Can you work these out from the model? Positions are in its coordinate system, mm. Give positions to 0.01 mm unless a question says otherwise; leave off trailing zeros. Order: outer loops, then holes, each group sorted by start corner. A loop starts at its lowest first (then second) coordinate and runs counter-clockwise, first axis right, second up. Notation, with made-up numbers: M 42.5,-25.75 L 48.5,-25.75 A38 cw 48.5,13.25 Z; hole C 41,66 d11. An arc over 180 degrees is marked long. One line per question, with ' | ' between items. Start each with the question number.
1) If we section it at A-A, the plane x = 0: Please give me the cut outline in (y, z).
2) I'm going to push flat-ended pins straight in: pin 1 Ø2 at (x, z) = (24.5, -180) entering from -Y; pin 2 Ø1.5 at (x, y) = (-2.5, 82) entering from -Z; pin 3 Ø12 at (x, y) = (24, -4) entering from +Z. Where does each tip first touch, or does it pass through?
3) If we section it at C-C, the plane y = -13.5: Please give me the cut outline in (x, z), plus the area to 3 significant figures.
4) Please list where these lines run through material, in increasing order: line 1 along Y through (x, z) = (11.5, -65) (3 decimals); line 2 along Y through (x, z) = (-6, -88); line 3 along Z through (x, y) = (5.5, 12). Write a range as [from, to].
5) If we section it at B-B, the plane z = -207.5: Please give me the cut outline in (x, y), plus the area to 3 significant figures.
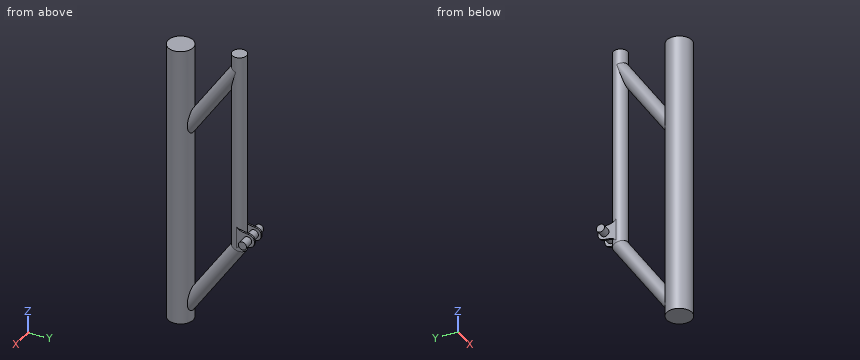
```python
from build123d import *

# Parameters (mm, degrees)
SKETCH1_R                = 25.8
BOSS_EXTRUDE1_DEPTH      = 544
SKETCH6_R                = 14.6
BOSS_EXTRUDE2_REACH      = 541.822
BOSS_EXTRUDE2_END_RADIUS = 25.8
SKETCH4_R                = 14.6
BOSS_EXTRUDE3_START      = -3.5
BOSS_EXTRUDE3_OUTLINE_R  = 8.35
BOSS_EXTRUDE3_DEPTH      = 3.5
BOSS_EXTRUDE4_START      = 17
SKETCH7_3_R              = 8.35
BOSS_EXTRUDE4_DEPTH      = 66
SKETCH9_R                = 25.8
BOSS_EXTRUDE5_DEPTH      = 16.49
BOSS_EXTRUDE6_START      = 23.51
SKETCH10_R               = 25.8
BOSS_EXTRUDE6_DEPTH      = 23.51
BOSS_EXTRUDE7_START      = 13
SKETCH11_R               = 14.6
BOSS_EXTRUDE7_DEPTH      = 13


# Read off the part's stored shape, not the designer's step: Boss-Extrude3
with BuildPart() as part:
    # Sketch1 → Boss-Extrude1 (new body)
    with BuildSketch(Plane.XY):
        Circle(SKETCH1_R)
    extrude(amount=-BOSS_EXTRUDE1_DEPTH)

    # Sweep2: sweep along a path in Sketch2
    with BuildLine(Plane(origin=(0, 0, 0), x_dir=(0, 0, -1), z_dir=(1, 0, 0))) as sweep2_path:
        Line((535.242725219, 10.616416132), (373.485286901, 119.6))
        Line((373.485286901, 119.6), (-26.514713099, 119.6))
    # Sketch6 → Sweep2 (sweep)
    with BuildSketch(Plane(origin=(0, 10.616416132, -535.242725219), x_dir=(1, 0, 0), z_dir=(0, 0.5587587437797145, 0.8293302516185669))):
        Circle(SKETCH6_R)
    sweep(path=sweep2_path.line, transition=Transition.RIGHT)

    # Boss-Extrude2: up to this cylinder (the profile starts outside it)
    boss_extrude2_end = Plane(origin=(0, 0, 7.489761), z_dir=(0, 0, 1)) * Cylinder(BOSS_EXTRUDE2_END_RADIUS, 1136.244, mode=Mode.PRIVATE)
    # Sketch4 → Boss-Extrude2 (add, up to the surface)
    with BuildSketch(Plane(origin=(0, 296.142134203, -111.454966642), x_dir=(1, 0, 0), z_dir=(0, 0.5587587437797145, 0.8293302516185669)), mode=Mode.PRIVATE) as boss_extrude2_sk1:
        with Locations(Location((0, -212.87313933, 0), (0, 0, 270))):
            Circle(SKETCH4_R)
    boss_extrude2_tool1 = extrude(boss_extrude2_sk1.sketch, amount=-BOSS_EXTRUDE2_REACH, mode=Mode.PRIVATE) - boss_extrude2_end
    add(boss_extrude2_tool1.solids().sort_by_distance((0, 119.6, 7.489761))[0])

    # Boss-Extrude3 outline → Boss-Extrude3 (add)
    with BuildSketch(Plane.ZY.offset(14.6).offset(BOSS_EXTRUDE3_START)):
        with BuildLine():
            add(Edge.make_bspline(
                [(-369.025798161, 121.314868638), (-354.153662916, 130.263805611), (-368.24558028, 157.483504956), (-346.0257981, 157.599948143)],
                knots=[0, 0, 0, 0, 0.999846057, 0.999846057, 0.999846057, 0.999846057], degree=3))
            Line((-369.025798161, 121.314868638), (-323.025798161, 121.314868638))
            add(Edge.make_bspline(
                [(-323.025798161, 121.314868638), (-337.897933379, 130.263805595), (-323.806016093, 157.483504857), (-346.0257981, 157.599948143)],
                knots=[0, 0, 0, 0, 0.999846056, 0.999846056, 0.999846056, 0.999846056], degree=3))
        make_face()
        with Locations((-346.025798161, 143.65)):
            Circle(BOSS_EXTRUDE3_OUTLINE_R, mode=Mode.SUBTRACT)
    boss_extrude3 = extrude(amount=BOSS_EXTRUDE3_DEPTH)

    # Mirror1: Boss-Extrude3 across plane
    add(boss_extrude3.mirror(Plane.ZY))

    # Sketch7<3> → Boss-Extrude4 (add)
    with BuildSketch(Plane.ZY.offset(14.6).offset(BOSS_EXTRUDE4_START)):
        with Locations((-346.025798161, 143.65)):
            Circle(SKETCH7_3_R)
    extrude(amount=-BOSS_EXTRUDE4_DEPTH)

    # Sketch9 → Boss-Extrude5 (add)
    with BuildSketch(Plane(origin=(0, 0, -544), x_dir=(-1, 0, 0), z_dir=(0, 0, -1))):
        with Locations(Location((0, 0, 0), (0, 0, 180))):
            Circle(SKETCH9_R)
    extrude(amount=BOSS_EXTRUDE5_DEPTH)

    # Sketch10 → Boss-Extrude6 (add)
    with BuildSketch(Plane.XY.offset(BOSS_EXTRUDE6_START)):
        Circle(SKETCH10_R)
    extrude(amount=-BOSS_EXTRUDE6_DEPTH)

    # Sketch11 → Boss-Extrude7 (add)
    with BuildSketch(Plane.XY.offset(26.514713099).offset(BOSS_EXTRUDE7_START)):
        with Locations((0, 119.6)):
            Circle(SKETCH11_R)
    extrude(amount=-BOSS_EXTRUDE7_DEPTH)


solid = part.part
```
Results found:
1) outline: M -25.8,-560.49 L 25.8,-560.49 L 25.8,-538.84 L 134.2,-377.94 L 134.2,39.51 L 105,39.51 L 105,11.95 L 25.8,-105.6 L 25.8,23.51 L -25.8,23.51 Z; C 143.65,-346.03 d16.7; hole M 25.8,-486.58 L 105,-369.03 L 105,-40.31 L 25.8,-157.86 Z
2) pin 1: stops at y = -10.65 | pin 2: stops at z = -456.17 | pin 3: stops at z = 23.51
3) outline: M -21.99,-560.49 L 21.99,-560.49 L 21.99,23.51 L -21.99,23.51 Z | area: 25,700 mm²
4) line 1: y = [-23.095, 23.095], [59.914, 81.606], [110.605, 128.595] | line 2: y = [-25.09, 25.09], [39.21, 71.31], [106.29, 132.91] | line 3: z = [-560.49, 23.51]
5) outline: C 0,0 d51.6; C 0,119.6 d29.2 | area: 2,760 mm²
